For this review, take the finished solid that the model builds, in its own axes (mm). A direction names the side the tool comes from. Coordinates: 2 decimals unless noted, no trailing zeros. Order: outer loops, then holes, each group sorted by start corner. A loop starts at its lowest first (then second) coordinate and runs counter-clockwise, first axis right, second up.
from build123d import *

# Parameters (mm, degrees)
CROQUIS2_W              = 200
CROQUIS2_H              = 150
CROQUIS2_R              = 2
CROQUIS2_R_2            = 2.5
CROQUIS2_W_2            = 31.297292299
CROQUIS2_H_2            = 43.768728426
CROQUIS2_H_3            = 43.768728427
CROQUIS2_W_3            = 23.573907934
CROQUIS2_H_4            = 45.323962431
SALIENTE_EXTRUIR1_DEPTH = 2
REDONDEO1_R             = 10
BOSS_EXTRUDE1_DEPTH     = 25
SKETCH3_W               = 62.040442094
SKETCH3_H               = 5.530821024
BOSS_EXTRUDE2_DEPTH     = 22
SKETCH8_W               = 62.040442094
SKETCH8_H               = 5.530821024
BOSS_EXTRUDE6_DEPTH     = 13
SKETCH2_W               = 200
SKETCH2_H               = 78.124132015
SKETCH2_W_2             = 62.040442094
SKETCH2_H_2             = 5.530821024
BOSS_EXTRUDE3_DEPTH     = 5
SKETCH4_W               = 62.040442094
SKETCH4_H               = 5.530821024
BOSS_EXTRUDE4_DEPTH     = 19
SKETCH5_W               = 7.442573222
SKETCH5_H               = 2.991451355
BOSS_EXTRUDE5_DEPTH     = 21
SKETCH6_R               = 2.5
CUT_EXTRUDE1_DEPTH      = 158.961544101
FILLET1_R               = 10
SKETCH10_W              = 79.68896036
SKETCH10_H              = 141.741238344
BOSS_EXTRUDE7_DEPTH     = 5
SKETCH11_W              = 5
SKETCH11_H              = 20
BOSS_EXTRUDE13_DEPTH    = 15
FILLET2_R               = 5
CUT_EXTRUDE3_DEPTH      = 215.07420719
SKETCH15_W              = 7
SKETCH15_H              = 40
CUT_EXTRUDE5_DEPTH      = 10
CROQUIS4_R              = 8.45
CROQUIS4_W              = 5.32
CROQUIS4_H              = 11.08
CORTAR_EXTRUIR3_DEPTH   = 95


# Read off the part's stored shape, not the designer's step: Cut-Extrude4
# Some blends are built 0.0001 mm under size
with BuildPart() as part:
    # Croquis2 → Saliente-Extruir1 (new body)
    with BuildSketch(Plane.XY):
        with Locations((0.108263467, -0.36008145)):
            Rectangle(CROQUIS2_W, CROQUIS2_H)
        with Locations((89.108263467, -66.5)):
            Circle(CROQUIS2_R, mode=Mode.SUBTRACT)
        with Locations((-88.891736533, -66.5)):
            Circle(CROQUIS2_R, mode=Mode.SUBTRACT)
        with Locations(Location((89.108263467, 65.779837101, 0), (0, 0, 180))):
            Circle(CROQUIS2_R, mode=Mode.SUBTRACT)
        with Locations(Location((-88.891736533, 65.779837101, 0), (0, 0, 180))):
            Circle(CROQUIS2_R, mode=Mode.SUBTRACT)
        with Locations((-80.865436179, -59.36008145)):
            Circle(CROQUIS2_R_2, mode=Mode.SUBTRACT)
        with Locations((81.108263467, -59.36008145)):
            Circle(CROQUIS2_R_2, mode=Mode.SUBTRACT)
        with Locations(Location((81.108263467, 58.63991855, 0), (0, 0, 180))):
            Circle(CROQUIS2_R_2, mode=Mode.SUBTRACT)
        with Locations(Location((-80.865436179, 58.63991855, 0), (0, 0, 180))):
            Circle(CROQUIS2_R_2, mode=Mode.SUBTRACT)
        with BuildLine():
            Line((-62.091736533, 70.63991855), (64.108263467, 70.63991855))
            ThreePointArc((64.108263467, 70.63991855), (66.108263467, 68.63991855), (64.108263467, 66.63991855))
            Line((64.108263467, 66.63991855), (-62.091736533, 66.63991855))
            ThreePointArc((-62.091736533, 66.63991855), (-64.091736533, 68.63991855), (-62.091736533, 70.63991855))
        make_face(mode=Mode.SUBTRACT)
        Polygon((-71.391736533, -12.902447307), (-71.391736533, 12.182284408), (-79.241736533, 12.28991855), (-83.891736533, 12.28991855), (-83.891736533, -13.01008145), (-79.241736533, -13.01008145), align=None, mode=Mode.SUBTRACT)
        with BuildLine():
            Line((92.108263467, 45.478381757), (92.108263467, -46.198544657))
            ThreePointArc((92.108263467, -46.198544657), (90.807295546, -47.897576736), (89.108263467, -46.596608814))
            Line((89.108263467, -46.596608814), (89.108263467, 45.876445915))
            ThreePointArc((89.108263467, 45.876445915), (90.807295546, 47.177413836), (92.108263467, 45.478381757))
        make_face(mode=Mode.SUBTRACT)
        Polygon((84.108263467, 12.28991855), (84.108263467, -13.01008145), (79.458263467, -13.01008145), (71.608263467, -13.01008145), (71.608263467, 12.28991855), (79.458263467, 12.28991855), align=None, mode=Mode.SUBTRACT)
        with BuildLine():
            Line((-91.891736533, 45.478381757), (-91.891736533, -46.198544657))
            ThreePointArc((-91.891736533, -46.198544657), (-90.590768612, -47.897576736), (-88.891736533, -46.596608814))
            Line((-88.891736533, -46.596608814), (-88.891736533, 45.876445915))
            ThreePointArc((-88.891736533, 45.876445915), (-90.590768612, 47.177413836), (-91.891736533, 45.478381757))
        make_face(mode=Mode.SUBTRACT)
        with Locations((-30.011405388, 36.299005811)):
            Rectangle(CROQUIS2_W_2, CROQUIS2_H_2, mode=Mode.SUBTRACT)
        with BuildLine():
            Line((-62.091736533, -71.36008145), (64.108263467, -71.36008145))
            ThreePointArc((64.108263467, -71.36008145), (66.108263467, -69.36008145), (64.108263467, -67.36008145))
            Line((64.108263467, -67.36008145), (-62.091736533, -67.36008145))
            ThreePointArc((-62.091736533, -67.36008145), (-64.091736533, -69.36008145), (-62.091736533, -71.36008145))
        make_face(mode=Mode.SUBTRACT)
        with Locations((-30.011405388, -26.799059535)):
            Rectangle(CROQUIS2_W_2, CROQUIS2_H_3, mode=Mode.SUBTRACT)
        with Locations((12.982877294, -0.693345879)):
            Rectangle(CROQUIS2_W_3, CROQUIS2_H_4, mode=Mode.SUBTRACT)
    extrude(amount=SALIENTE_EXTRUIR1_DEPTH)

    # Redondeo1
    redondeo1_edges = [part.edges().sort_by_distance(p)[0] for p in [
        (100.108263467, -75.36008145, 1),
        (-99.891736533, -75.36008145, 1),
        (-99.891736533, 74.63991855, 1),
        (100.108263467, 74.63991855, 1),
    ]]
    fillet(redondeo1_edges, radius=REDONDEO1_R)

    # Sketch1 → Boss-Extrude1 (add)
    with BuildSketch(Plane.XY.offset(2)):
        Polygon((-67.071845217, 64.63991855), (-67.071845217, 60.63991855), (-8.841198185, 60.63991855), (-8.841198185, 3.63991855), (-67.071845217, 3.63991855), (-67.071845217, -0.36008145), (-8.841198185, -0.36008145), (-8.841198185, -53.36008145), (-67.071845217, -53.36008145), (-67.071845217, -57.574734434), (-5.031403123, -57.574734434), (-5.031403123, -40.931443482), (46.608263467, -40.931443482), (46.608263467, -36.931443482), (-5.031403123, -36.931443482), (-5.031403123, 30.068556518), (46.608263467, 30.068556518), (46.608263467, 34.068556518), (-5.031403123, 34.068556518), (-5.031403123, 64.63991855), align=None)
    extrude(amount=BOSS_EXTRUDE1_DEPTH)

    # Sketch3 → Boss-Extrude2 (add)
    with BuildSketch(Plane.XZ.offset(57.574734434)):
        with Locations((-36.05162417, 24.234589488)):
            Rectangle(SKETCH3_W, SKETCH3_H)
    extrude(amount=BOSS_EXTRUDE2_DEPTH)

    # Sketch8 → Boss-Extrude6 (add)
    with BuildSketch(Plane(origin=(0, 64.63991855, 0), x_dir=(1, 0, 0), z_dir=(0, 1, 0))):
        with Locations((-36.05162417, -24.234589488)):
            Rectangle(SKETCH8_W, SKETCH8_H)
    extrude(amount=BOSS_EXTRUDE6_DEPTH)

    # Sketch2 → Boss-Extrude3 (add)
    with BuildSketch(Plane.XZ.offset(75.36008145)):
        with Locations((0.108263467, 41.062066008)):
            Rectangle(SKETCH2_W, SKETCH2_H)
        with Locations((-36.05162417, 24.234589488)):
            Rectangle(SKETCH2_W_2, SKETCH2_H_2, mode=Mode.SUBTRACT)
    extrude(amount=-BOSS_EXTRUDE3_DEPTH)

    # Sketch4 → Boss-Extrude4 (add)
    with BuildSketch(Plane(origin=(0, 64.63991855, 0), x_dir=(1, 0, 0), z_dir=(0, 1, 0))):
        with Locations((-36.05162417, -24.234589488)):
            Rectangle(SKETCH4_W, SKETCH4_H)
    extrude(amount=BOSS_EXTRUDE4_DEPTH)

    # Sketch5 → Boss-Extrude5 (add)
    with BuildSketch(Plane.XZ.offset(75.36008145)):
        with Locations((-80.540187187, 3.495725678)):
            Rectangle(SKETCH5_W, SKETCH5_H)
        with Locations((80.756714122, 3.495725678)):
            Rectangle(SKETCH5_W, SKETCH5_H)
    extrude(amount=BOSS_EXTRUDE5_DEPTH)

    # Sketch6 → Cut-Extrude1 (cut, through all)
    with BuildSketch(Plane.XY.offset(4.991451355)):
        with Locations((-80.996023003, -59.284349751)):
            Circle(SKETCH6_R)
        with Locations((81.166025964, -59.051385225)):
            Circle(SKETCH6_R)
    extrude(amount=-CUT_EXTRUDE1_DEPTH, mode=Mode.SUBTRACT)

    # Fillet1
    # the kernel refuses this fillet: 10 mm, written as the material it takes off along each edge
    with BuildSketch(Plane(origin=(100.108263467, -70.36008145, 2), x_dir=(-1, 0, 0), z_dir=(0, 0, 1)), Plane(origin=(-99.891736533, -70.36008145, 101.77476711), x_dir=(1, 0, 0), z_dir=(0, 0, -1))) as fillet1_piece_1:
        with BuildLine():
            CenterArc((8.660254038, 10), FILLET1_R, 210, 60)
            Line((0, 5), (0, 0))
            Line((0, 0), (8.660254038, 0))
        make_face()
    extrude(amount=99.77476711, mode=Mode.SUBTRACT)


with BuildPart() as body_2:
    # Sketch10 → Boss-Extrude7 (new body)
    with BuildSketch(Plane.ZY.offset(99.891736533)):
        with Locations((-39.84448018, -2.473210197)):
            Rectangle(SKETCH10_W, SKETCH10_H)
    extrude(amount=BOSS_EXTRUDE7_DEPTH)

    # Sketch11 → Boss-Extrude13 (add)
    with BuildSketch(Plane.ZY.offset(104.891736533)):
        with Locations((-2.5, -53.343829369)):
            Rectangle(SKETCH11_W, SKETCH11_H)
        with Locations((-2.5, 48.397408975)):
            Rectangle(SKETCH11_W, SKETCH11_H)
    extrude(amount=-BOSS_EXTRUDE13_DEPTH)

    # Fillet2
    fillet2_edges = [body_2.edges().sort_by_distance(p)[0] for p in [
        (-104.891736533, 68.397408975, -39.84448018),
        (-104.891736533, -73.343829369, -39.84448018),
    ]]
    fillet(fillet2_edges, radius=FILLET2_R - 0.0001)  # a hair under: the kernel refuses the full size


with BuildPart() as cut_extrude3_tool:
    # Sketch13 → Cut-Extrude3 (new, through all)
    with BuildSketch(Plane.XY.offset(80.124132015)):
        Polygon((-88.891736533, 38.397408975), (-87.891736533, 38.397408975), (-87.891736533, 63.52554782), (-99.891736533, 63.52554782), (-99.891736533, 94.010082764), (108.48763668, 94.010082764), (108.48763668, -102.123784964), (-99.891736533, -102.123784964), (-99.891736533, -61.922986139), (-88.478309969, -61.922986139), (-88.478309969, -40.956005085), (-99.891736533, -40.956005085), (-99.891736533, 38.397408975), align=None)
    extrude(amount=-CUT_EXTRUDE3_DEPTH)


with BuildPart() as part_1:
    add(part.part)

    # Cut-Extrude3: cut by cut_extrude3_tool
    add(cut_extrude3_tool.part, mode=Mode.SUBTRACT)


with BuildPart() as body_2_1:
    add(body_2.part)

    # Cut-Extrude3: cut by cut_extrude3_tool
    add(cut_extrude3_tool.part, mode=Mode.SUBTRACT)

    # Sketch15 → Cut-Extrude5 (cut)
    with BuildSketch(Plane(origin=(-99.891736533, 0, 0), x_dir=(0, 0, -1), z_dir=(1, 0, 0))):
        with Locations((76.18896036, 0)):
            Rectangle(SKETCH15_W, SKETCH15_H)
    extrude(amount=-CUT_EXTRUDE5_DEPTH, mode=Mode.SUBTRACT)

    # Croquis4 → Cortar-Extruir3 (cut)
    with BuildSketch(Plane.ZY.offset(104.891736533)):
        with Locations((-13, 10.526789803)):
            Circle(CROQUIS4_R)
        with Locations((-13, -15.473210197)):
            Circle(CROQUIS4_R)
        with Locations((-20.34, -2.473210197)):
            Rectangle(CROQUIS4_W, CROQUIS4_H)
    extrude(amount=-CORTAR_EXTRUIR3_DEPTH, mode=Mode.SUBTRACT)


solid = body_2_1.part
1. Take a section at B-B, the plane x = -94.25. Give the boundary of the cut face in (y, z).
Answer below:
outline: (-61.92, -5) - (-43.34, -5) - (-43.34, 0) - (-61.92, 0) - close; (38.4, -5) - (58.4, -5) - (58.4, 0) - (38.4, 0) - close
2. The part is to be moulded in two halves that separate along Z. For faces 6 (the face through (-95, -53, -5)), 7 (the face through (-102, -3, -17.68)), 8 (the face through (-89.892, -53, -3)), say which applies: +Z half, -Z half, draft (parallel to the pull), parting line (faces both ways), or undercut.
Answer below:
face 6: -Z half
face 7: undercut
face 8: draft
3. Clearance check with flat-ended pins moving along their axes: pin 1 Ø4 at (x, z) = (-96, -22.5) entering from +Y; pin 2 Ø3 at (x, y) = (-101, -6.5) entering from -Z; pin 3 Ø4 at (y, z) = (-55.5, -21.5) entering from +X; pin 4 Ø5.5 at (x, z) = (-94.5, -2.5) entering from -Y. State where each tip first meets the part, or that it passes through.
Answer below:
pin 1: passes through
pin 2: stops at z = -72.69
pin 3: stops at x = -99.89
pin 4: stops at y = -61.92
4. To check wall thickness, follow L1, parallel to Y at x = -92, z = -4.5; L2, parallel to Y at x = -101.45, z = -13; L3, parallel to Y at x = -102.35, z = -13. State the ranges of each line that lie inside material, in increasing order.
Answer below:
L1: y = -61.92 to -43.34, 38.4 to 58.4
L2: y = -73.09 to -23.92, -7.02 to 2.08, 18.98 to 68.15
L3: y = -72.7 to -23.92, -7.02 to 2.08, 18.98 to 67.75
5. Machinability: for faces 1 (the face through (-95, 38.397, -3)), 2 (the face through (-102, -8.013, -20)), 3 (the face through (-102, 0, -72.689)), 4 (the face through (-95, 48, -5)), 5 (the face through (-95, -61.923, -2)), which of the approach directions +Z, -Z, +X, -X, +Y, -Y give a long, thin tool a straight path to every point of the face, cutting with its end or side? Answer none if there is none.
Answer below:
face 1: +Z, -Z, +X
face 2: +X, -X
face 3: -Z, +X, -X
face 4: -Z, +X, +Y, -Y
face 5: +Z, -Z, +X, -Y
6. Take a section at A-A, the plane z = -13. Give the number of separate pieces and of enclosed holes in the cut face, plus the area to 3 significant figures.
Answer below:
separate pieces: 3
enclosed holes: 0
area: 529 mm2
7. Take a section at D-D, the plane x = -101.75. Give the boundary of the cut face in (y, z).
Answer below:
outline: (-72.99, -79.69) - (-20, -79.69) - (-20, -72.69) - (20, -72.69) - (20, -79.69) - (68.04, -79.69) - (68.04, 0) - (-72.99, 0) - close; hole circle Ø16.9 at (-15.47, -13); hole (-8.01, -23) - (3.07, -23) - (3.07, -17.68) - (-8.01, -17.68) - close; hole circle Ø16.9 at (10.53, -13)
